Geometry check sheet. Reference: the model listing, model coordinates, mm. Face numbers are marked on the shaded views. Round coordinates to 2 decimals unless told otherwise and drop trailing zeros. Write each loop counter-clockwise with the first axis right and the second up, starting at its lowest first coordinate (ties: lowest second). Pieces come first, ordered by that corner, then holes. Notation, with made-up numbers: M -16.75,-22 L -6.75,-22 A31 ccw -6.75,12 Z; hole C -27,-30 d2. An arc over 180 degrees is marked long. One line per item, written item: value. Start each with the question number.
1. Section check C-C (z = 106.5). Record the boundary of the cut face in (x, y), and give its area (3 significant figures).
2. Scan lines: probe 1 along Z at (x, y) = (-138.75, -20); probe 2 along Z at (x, y) = (-143, -20); probe 3 along X at (y, z) = (-34.5, -16.5). Record each from-to range of solid material in increasing order. Write a range as [from, to].
3. Release check for a two-part mould opening along Y. For the marked faces 1 and 2 record: pulls with the +Y half, pulls with the -Y half, needs draft (parallel to the pull), parting line crosses it, or undercut.
4. Section check A-A (y = -20). Record the boundary of the cut face in (x, z), and give its area (3 significant figures).
5. Depth check by flat-ended pin: P1, Ø12, axis at y = -28, z = 126, coming from the -X side; P2, Ø2, axis at x = 9.5, y = -34.5, coming from the -Z side; P3, Ø6, axis at y = -27, z = 137, coming from the -X side. Enter the tip coordinate at first touch or a pass-through.
6. Section check B-B (x = -99.5). Record the boundary of the cut face in (y, z), and give its area (3 significant figures).
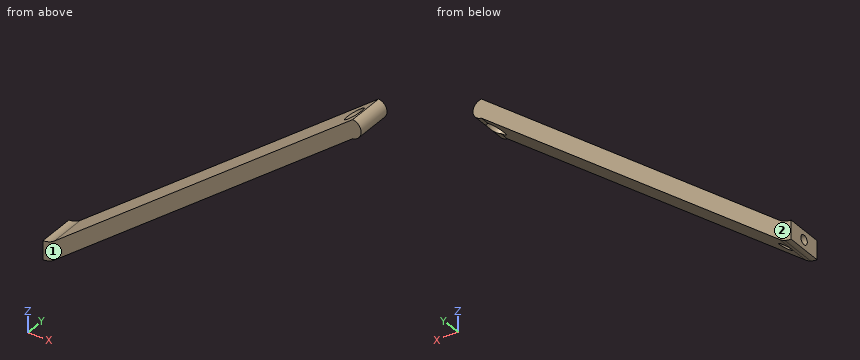
from build123d import *

# Parameters (mm, degrees)
F1_DEPTH = 40
F3_D     = 10
F5_D     = 20


with BuildPart() as f1:
    # F0 (on Front) → F1 (new body)
    with BuildSketch(Plane.XZ):
        with BuildLine():
            ThreePointArc((-138.652626, -5.954697), (-144.411955, -9.044339), (-150.859851, -10.112232))
            Line((-150.859851, -10.112232), (-150.859851, -30.112232))
            ThreePointArc((-150.859851, -30.112232), (-147.401977, -29.811042), (-144.048252, -28.916544))
            ThreePointArc((-144.048252, -28.916544), (-141.235816, -27.64443), (-138.652626, -25.954697))
            Line((-138.652626, -25.954697), (178.3398, 218.300084))
            ThreePointArc((178.3398, 218.300084), (187.221678, 228.309372), (178.19666, 238.189789))
            Line((178.19666, 238.189789), (-138.652626, -5.954697))
        make_face()
    extrude(amount=F1_DEPTH)

    # F3 (through all)
    with Locations(Plane(origin=(-150.859851, 0, 0), x_dir=(0, -1, 0), z_dir=(-1, 0, 0))):
        with Locations((20, -20.112232)):
            Hole(F3_D / 2)

    # F5 (through all)
    with Locations(Plane(origin=(-48.774778, 0, 63.299621), x_dir=(0.792123, 0, 0.610361), z_dir=(-0.610361, 0, 0.792123))):
        with Locations((271.53552, -20)):
            Hole(F5_D / 2)


solid = f1.part
Result sheet:
1. outline: M 7.29,-40 L 33.25,-40 L 33.25,0 L 7.29,0 Z
1. area: 1,040 mm2
2. probe 1: z = [-26.03, -25.11], [-15.11, -6.03]
2. probe 2: z = [-28.5, -25.11], [-15.11, -8.5]
2. probe 3: x = [-150.86, -126.38]
3. face 1: pulls with the -Y half
3. face 2: pulls with the +Y half
4. outline: M -150.86,-30.11 A20 ccw -144.05,-28.92 A20 ccw -138.65,-25.95 L -137.56,-25.11 L -150.86,-25.11 Z; M -150.86,-15.11 L -124.58,-15.11 L 168.06,210.38 L 158.39,222.93 L -138.65,-5.95 A20 cw -150.86,-10.11 Z; M 174.24,235.14 L 184.68,221.58 A10 ccw 178.2,238.19 Z
4. area: 6,200 mm2
5. P1: stops at x = 24.81
5. P2: stops at z = 87.43
5. P3: stops at x = 42.98
6. outline: M -40,4.21 L 0,4.21 L 0,24.21 L -40,24.21 Z
6. area: 800 mm2
